Here's the drawing with two shaded views (mm, measured from the low corner). I have some questions. A direction names the side the tool comes from. Coordinates: 2 decimals unless noted, no trailing zeros. Write each loop counter-clockwise with the first axis right and the second up, starting at its lowest first coordinate (ties: lowest second). Pieces come first, ordered by that corner, then holes. Notation, with made-up numbers: (-20, 40.25) -> (-3, 40.25) arc R20 ccw to (-3, 49.25) -> close; hole circle Ø7 at (72.25, 0.25). An arc over 180 degrees is marked (long way). Use one line per item in the form item = value.
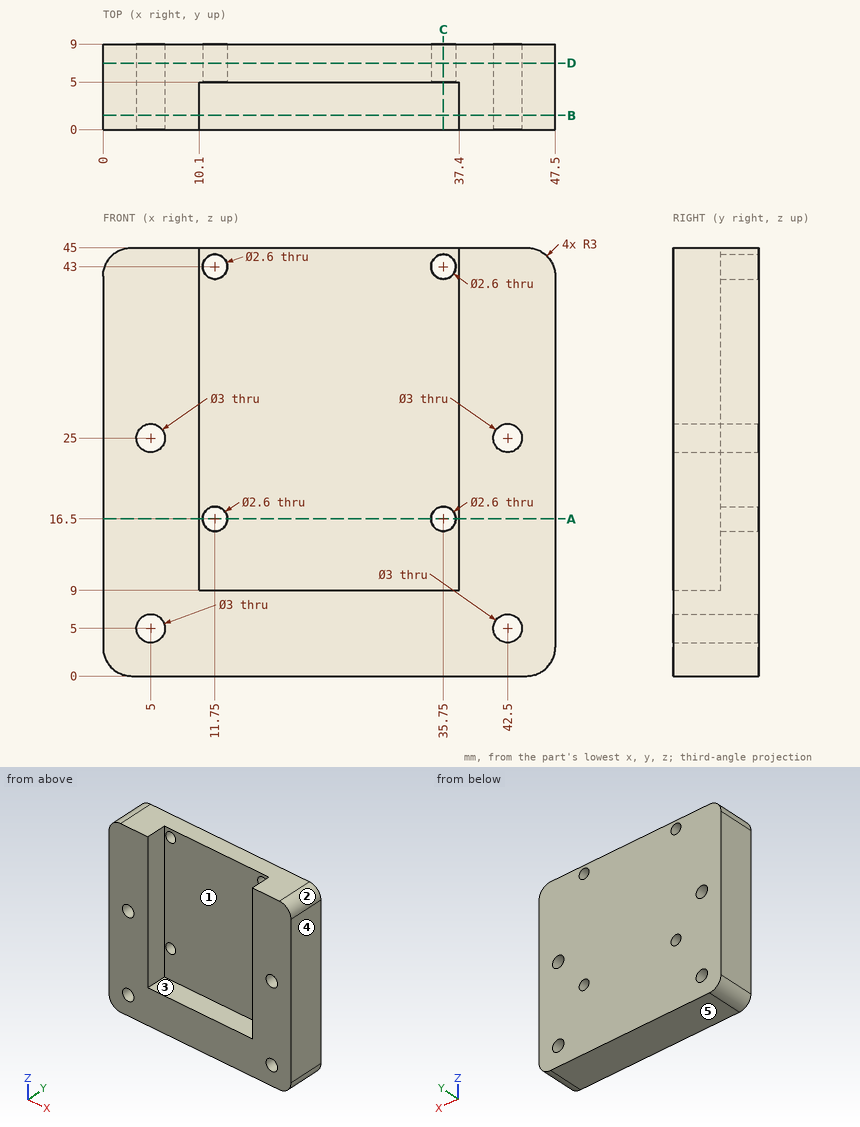
Q1. Suppose I cut it at D-D (y = 7). Give the number of separate pieces and of enclosed holes in the cut face, then the cut area to 3 significant figures.
Return value:
separate_pieces = 1
enclosed_holes = 8
area = 2,080 mm2
Q2. If I drill on line 1 (X direction, y = 6.8, z = 16.5); line 2 (Z direction, x = 42.5, y = 5.75); line 3 (X direction, y = 4.5, z = 15.5), over which ranges is the centre line in solid material (lowest first)? Write a range as from..to.
Return value:
line_1 = 0..10.45, 13.05..34.45, 37.05..47.5
line_2 = 0..3.5, 6.5..23.5, 26.5..45
line_3 = 0..10.1, 37.4..47.5
Q3. Suppose I cut it at A-A (z = 16.5). Write out the boundary of the cut face in (x, y), then the cut area to 3 significant figures.
Return value:
outline = (0, 0) -> (10.1, 0) -> (10.1, 5) -> (10.45, 5) -> (10.45, 9) -> (0, 9) -> close; (13.05, 5) -> (34.45, 5) -> (34.45, 9) -> (13.05, 9) -> close; (37.05, 5) -> (37.4, 5) -> (37.4, 0) -> (47.5, 0) -> (47.5, 9) -> (37.05, 9) -> close
area = 270 mm2
Q4. For the marked faces 1 and 2, which set-ups out of +Z, -Z, +X, -X, +Y, -Y let a thin tool reach every point of the face, with its end or its side?
Return value:
face_1 = +Z, -Y
face_2 = +Z, +X, +Y, -Y
Q5. Thinking about a two-plate mould opening in X: for the marked faces 3, 4 and 5, which applies, released by +X, released by -X, zero draft, split by the parting line, or undercut?
Return value:
face_3 = undercut
face_4 = released by +X
face_5 = zero draft
Q6. Suppose I cut it at B-B (y = 1.5). Write out the boundary of the cut face in (x, z), then the cut area to 3 significant figures.
Return value:
outline = (0, 3) arc R3 ccw to (3, 0) -> (44.5, 0) arc R3 ccw to (47.5, 3) -> (47.5, 42) arc R3 ccw to (44.5, 45) -> (37.4, 45) -> (37.4, 9) -> (10.1, 9) -> (10.1, 45) -> (3, 45) arc R3 ccw to (0, 42) -> close; hole circle Ø3 at (5, 5); hole circle Ø3 at (5, 25); hole circle Ø3 at (42.5, 5); hole circle Ø3 at (42.5, 25)
area = 1,120 mm2
Q7. Will these pins go through, and if not, where does the flat tip stop? pin 1 (3 mm diameter, centred on x = 27, z = 34, fed in from -Y); pin 2 (1.5 mm diameter, centred on x = 15, y = 2, fed in from +Z).
Return value:
pin_1 = 5
pin_2 = 9
Q8. Suppose I cut it at C-C (x = 35.75). Write out the boundary of the cut face in (y, z), then the cut area to 3 significant figures.
Return value:
outline = (0, 0) -> (9, 0) -> (9, 15.2) -> (5, 15.2) -> (5, 9) -> (0, 9) -> close; (5, 17.8) -> (9, 17.8) -> (9, 41.7) -> (5, 41.7) -> close; (5, 44.3) -> (9, 44.3) -> (9, 45) -> (5, 45) -> close
area = 204 mm2
